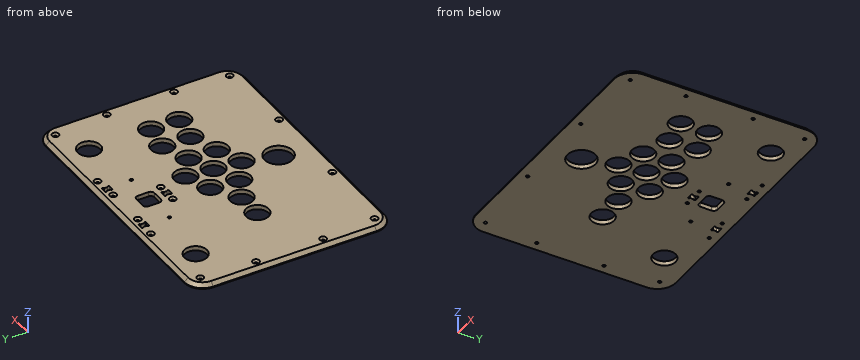
Autodesk Inventor part; units mm, degrees
ref_plane "YZ Plane" through (0, 0, 0) normal (1, 0, 0) x (0, 1, 0)
ref_plane "XZ Plane" through (0, 0, 0) normal (0, 1, 0) x (-1, 0, 0)
ref_plane "XY Plane" through (0, 0, 0) normal (0, 0, 1) x (1, 0, 0)
sketch "Sketch1" plane through (0, 0, 0) normal (0, 0, 1) x (1, 0, 0)
  line L0 (-150, 110) -> (150, 110)
  line L1 (150, 110) -> (150, -110)
  line L2 (150, -110) -> (-150, -110)
  line L3 (-150, -110) -> (-150, 110)
  line L4 (-150, 110) -> (150, -110) construction
  line L5 (150, 110) -> (-150, -110) construction
  point P0 (0, 0)
  dimension "d0" = 300
  dimension "d1" = 220
extrude "Extrusion1" add sketch "Sketch1" along normal blind 5
sketch "Sketch2" plane through (0, 0, 5) normal (0, 0, 1) x (1, 0, 0)
  line L0 (-150, -110) -> (150, -110)
  line L1 (9.7, -35) -> (14.9, 23.8) construction
  line L2 (-12.9, 12.8) -> (37.5, -24) construction
  line L3 (-100, 80) -> (100, 80) construction
  line L4 (150, 110) -> (-150, 110)
  line L5 (-150, 110) -> (-150, -110)
  arc A0 (9.7, -35) -> (-41.8, -4.7) centre (-117.4638, -192.22) ccw
  point P0 (0, 0)
  point P1 (0, -70)
  point P2 (-15.5, -17.6)
  point P3 (-71.3, -4.8)
  point P4 (12.3, -5.6)
  point P5 (39.2, 6.1)
  point P6 (68.8, -13.3)
  point P7 (68.8, 17.7)
  point P8 (98.3, -18.3)
  point P9 (98.3, 12.7)
  point P10 (12.3, -5.6)
  point P11 (0, 80)
  point P12 (-60, 80)
  point P13 (60, 80)
  point P14 (31.5334, -55.5137)
  point P15 (-14.9246, -17.9372)
  dimension "d4" = 40
  dimension "d5" = 15.5
  dimension "d6" = 26.3
  dimension "d7" = 29.5
  dimension "d11" = 52.4
  dimension "d12" = 65.3
  dimension "d13" = 65.2
  dimension "d14" = 9.7
  dimension "d15" = 29.4
  dimension "d16" = 2.6
  dimension "d17" = 26.9
  dimension "d18" = 29.6
  dimension "d19" = 29.5
  dimension "d20" = 1.7
  dimension "d22" = 46
  dimension "d23" = 30.1
  dimension "d24" = 96.7
  dimension "d25" = 91.7
  dimension "d26" = 31
  dimension "d27" = 31
  dimension "d28" = 35
  dimension "d61" = 30
  dimension "d62" = 50
  dimension "d63" = 8.496
  dimension "d64" = 8.496
  dimension "d65" = 40
  dimension "d66" = 40
hole "Hole1" at (0, -70, 5) at (-15.5, -17.6, 5) at (-41.8, -4.7, 5) at (-71.3, -4.8, 5) at (9.7, -35, 5) at (12.3, -5.6, 5) at (37.5, -24, 5) at (39.2, 6.1, 5) at (68.8, -13.3, 5) at (68.8, 17.7, 5) at (98.3, -18.3, 5) at (98.3, 12.7, 5) at (-12.9, 12.8, 5) at (14.9, 23.8, 5) at (-100, 80, 5) at (100, 80, 5) direction (0, 0, -1) diameter 25 end through all
sketch "Sketch5" plane through (0, 0, 5) normal (0, 0, 1) x (1, 0, 0)
  circle A0 centre (0, -70) radius 12.5
  point P0 (0, 0)
hole "Hole2" at (0, -70, 5) direction (0, 0, -1) diameter 31 end through all
sketch "Sketch6" plane through (0, 0, 5) normal (0, 0, 1) x (1, 0, 0)
  line L0 (-35.7, 71.2) -> (35.7, 71.2) construction
  line L1 (150, 110) -> (-150, 110)
  point P0 (0, 0)
  point P1 (0, 71.2)
  dimension "d67" = 71.4
  dimension "d68" = 38.8
hole "Hole3" at (-35.7, 71.2, 5) at (35.7, 71.2, 5) direction (0, 0, -1) diameter 3.4 end through all
fillet "Fillet2" radius 20 4 edges at (-150, 110, 2.5) (-150, -110, 2.5) (150, -110, 2.5) (150, 110, 2.5)
chamfer "Chamfer1" distance 4 angle 45 8 edges at (0, -110, 5) (144.1421, -104.1421, 5) (150, 0, 5) (144.1421, 104.1421, 5) (0, 110, 5) (-144.1421, 104.1421, 5) (-150, 0, 5) (-144.1421, -104.1421, 5)
sketch "Sketch8" plane through (0, 0, 5) normal (0, 0, 1) x (1, 0, 0)
  line L0 (130, 110) -> (-130, 110)
  line L1 (-150, 90) -> (-150, -90)
  line L2 (-130, -110) -> (130, -110)
  line L3 (150, -90) -> (150, 90)
  point P0 (0, 0)
  point P1 (-140, 37)
  point P2 (-50, 100)
  point P3 (-136, 96)
  dimension "d85" = 10
  dimension "d86" = 10
  dimension "d87" = 220
  dimension "d88" = 300
  dimension "d89" = 73
  dimension "d90" = 100
  dimension "d91" = 14
  dimension "d92" = 14
hole "Hole4" at (-140, 37, 5) at (-50, 100, 5) at (-136, 96, 5) direction (0, 0, -1) diameter 3.4 end through all countersink diameter 7.5 countersink angle 90
mirror "Mirror1" about plane through (0, 0, 0) normal (1, 0, 0) of "Hole4"
mirror "Mirror2" about plane through (0, 0, 0) normal (0, 1, 0) of "Hole4", "Mirror1"
sketch "Sketch9" plane through (0, 0, 5) normal (0, 0, 1) x (1, 0, 0)
  line L0 (-6, 83.2) -> (6, 83.2)
  line L1 (10, 79.2) -> (10, 67.2)
  line L2 (6, 63.2) -> (-6, 63.2)
  line L3 (-10, 67.2) -> (-10, 79.2)
  circle A0 centre (-35.7, 71.2) radius 1.7
  circle A1 centre (35.7, 71.2) radius 1.7
  line L4 (-35.7, 71.2) -> (35.7, 71.2) construction
  arc A2 (-6, 83.2) -> (-10, 79.2) centre (-6, 79.2) ccw
  arc A3 (10, 79.2) -> (6, 83.2) centre (6, 79.2) ccw
  arc A4 (-10, 67.2) -> (-6, 63.2) centre (-6, 67.2) ccw
  arc A5 (6, 63.2) -> (10, 67.2) centre (6, 67.2) ccw
  point P0 (0, 0)
  point P1 (-10, 83.2)
  point P2 (10, 63.2)
  point P3 (10, 83.2)
  point P4 (0, 83.2)
  point P5 (0, 71.2)
  point P6 (-10, 73.2)
  dimension "d100" = 20
  dimension "d101" = 20
  dimension "d102" = 2
  dimension "d103" = 4
extrude "Extrusion5" cut sketch "Sketch9" against normal through all contours L0 A3 L1 A5 L2 A4 L3 A2
sketch "Sketch10" plane through (0, 0, 5) normal (0, 0, 1) x (1, 0, 0)
  line L0 (-11.25, 53.2) -> (11.25, 53.2) construction
  circle A0 centre (35.7, 71.2) radius 1.7
  circle A1 centre (-35.7, 71.2) radius 1.7
  circle A2 centre (35.7, 71.2) radius 1.7
  line L1 (-35.7, 71.2) -> (35.7, 71.2) construction
  line L2 (0, 71.2) -> (0, 98.6) construction
  line L3 (-34.4, 98.6) -> (34.4, 98.6) construction
  line L4 (23.15, 98.6) -> (45.65, 98.6) construction
  line L5 (-45.65, 98.6) -> (-23.15, 98.6) construction
  point P0 (0, 0)
  point P1 (0, 53.2)
  dimension "d106" = 22.5
  dimension "d107" = 18
  dimension "d108" = 22.5
  dimension "d109" = 22.5
  dimension "d110" = 27.4
  dimension "d111" = 68.8
hole "Hole5" at (-11.25, 53.2, 5) at (11.25, 53.2, 5) at (23.15, 98.6, 5) at (-23.15, 98.6, 5) direction (0, 0, -1) diameter 3.4 end through all countersink diameter 7.5 countersink angle 90
sketch "Sketch11" plane through (0, 0, 5) normal (0, 0, 1) x (1, 0, 0)
  circle A0 centre (-11.25, 53.2) radius 1.7 construction
  circle A1 centre (11.25, 53.2) radius 1.7 construction
  line L0 (-11.25, 53.2) -> (11.25, 53.2) construction
  circle A2 centre (23.15, 98.6) radius 1.7 construction
  line L1 (23.15, 98.6) -> (45.65, 98.6) construction
  line L2 (-23.15, 98.6) -> (-45.65, 98.6) construction
  line L3 (-2.55, 49.15) -> (2.55, 49.15)
  line L4 (2.55, 49.15) -> (2.55, 57.25)
  line L5 (2.55, 57.25) -> (-2.55, 57.25)
  line L6 (-2.55, 57.25) -> (-2.55, 49.15)
  line L7 (-2.55, 49.15) -> (2.55, 57.25) construction
  line L8 (2.55, 49.15) -> (-2.55, 57.25) construction
  circle A3 centre (-2.55, 50.15) radius 1
  circle A4 centre (2.55, 50.15) radius 1
  circle A5 centre (2.55, 56.25) radius 1
  circle A6 centre (-2.55, 56.25) radius 1
  line L9 (-36.95, 94.55) -> (-31.85, 94.55)
  line L10 (-31.85, 94.55) -> (-31.85, 102.65)
  line L11 (-31.85, 102.65) -> (-36.95, 102.65)
  line L12 (-36.95, 102.65) -> (-36.95, 94.55)
  line L13 (-36.95, 94.55) -> (-31.85, 102.65) construction
  line L14 (-31.85, 94.55) -> (-36.95, 102.65) construction
  circle A7 centre (-36.95, 95.55) radius 1
  circle A8 centre (-31.85, 95.55) radius 1
  circle A9 centre (-31.85, 101.65) radius 1
  circle A10 centre (-36.95, 101.65) radius 1
  line L15 (31.85, 94.55) -> (36.95, 94.55)
  line L16 (36.95, 94.55) -> (36.95, 102.65)
  line L17 (36.95, 102.65) -> (31.85, 102.65)
  line L18 (31.85, 102.65) -> (31.85, 94.55)
  line L19 (31.85, 94.55) -> (36.95, 102.65) construction
  line L20 (36.95, 94.55) -> (31.85, 102.65) construction
  circle A11 centre (31.85, 95.55) radius 1
  circle A12 centre (36.95, 95.55) radius 1
  circle A13 centre (36.95, 101.65) radius 1
  circle A14 centre (31.85, 101.65) radius 1
  circle A15 centre (-23.15, 98.6) radius 1.7
  point P0 (0, 0)
  point P1 (0, 53.2)
  point P2 (-34.4, 98.6)
  point P3 (34.4, 98.6)
  point P4 (31.85, 100.65)
  point P5 (31.85, 96.55)
  point P6 (36.95, 96.55)
  point P7 (36.95, 100.65)
  point P8 (-31.85, 96.55)
  point P9 (-31.85, 100.65)
  point P10 (-36.95, 100.65)
  point P11 (-36.95, 96.55)
  point P12 (-2.55, 55.25)
  point P13 (-2.55, 51.15)
  point P14 (2.55, 51.15)
  point P15 (2.55, 55.25)
  dimension "d121" = 2
  dimension "d124" = 2
  dimension "d127" = 2
  dimension "d119" = 8.1
  dimension "d120" = 5.1
  dimension "d122" = 8.1
  dimension "d123" = 5.1
  dimension "d125" = 8.1
  dimension "d126" = 5.1
  dimension "d130" = 11.25
  dimension "d131" = 11.25
  dimension "d132" = 11.25
extrude "Extrusion6" cut sketch "Sketch11" against normal through all contours A3 L6 A6 L5 A5 L4 A4 L3 | A3 L6 | L6 A3 | A4 L4 | L4 A4 | A6 L6 | L6 A6 | A5 L4 | L4 A5 | A7 L12 A10 L11 A9 L10 A8 L9 | A7 L12 | L12 A7 | A8 L10 | L10 A8 | A10 L12 | L12 A10 | A9 L10 | L10 A9 | A11 L18 A14 L17 A13 L16 A12 L15 | A11 L18 | L18 A11 | A12 L16 | L16 A12 | A14 L18 | L18 A14 | A13 L16 | L16 A13
properties part number "Top Plate Sanwa" material "Polycarbonate, Clear"
Geometry: final body of the model. Coordinates: model frame, mm. Give positions to 0.01 mm unless a question says otherwise; leave off trailing zeros. Loops run counter-clockwise (first coordinate to the right, second up) from the corner with the lowest first, then second, coordinate; pieces in that order, holes last. Notation, with made-up numbers: (32, -38.75) -> (62, -38.75) arc R22 ccw to (62, -20.75) -> close; hole circle Ø3 at (-6.75, 9.5). An arc over 180 degrees is marked (long way). Use one line per item in the form item = value.
Item 1: Pin query (flat end, axial travel): P1, Ø1.5, axis at y = -47, z = 3, coming from the -X side; P2, Ø3, axis at x = -50, y = -100, coming from the +Z side; P3, Ø1.5, axis at x = 28, z = 2, coming from the +Y side; P4, Ø1.5, axis at x = -17.5, z = 4, coming from the +Y side. Return the tip coordinate at first contact, or that it passes through.
A:
P1 = -148.75
P2 = through
P3 = 109.75
P4 = 107.75
Item 2: Section query B-B on x = 92.5. Output: boundary loops of the cut face in (y, z).
A:
outline = (-110, 0) -> (-29.37, 0) -> (-29.37, 5) -> (-106, 5) -> (-110, 1) -> close; (-7.23, 0) -> (1.63, 0) -> (1.63, 5) -> (-7.23, 5) -> close; (23.77, 0) -> (70, 0) -> (70, 5) -> (23.77, 5) -> close; (90, 0) -> (110, 0) -> (110, 1) -> (106, 5) -> (90, 5) -> close
Item 3: Section query A-A on x = -41.8. Output: boundary loops of the cut face in (y, z), and give its area (3 significant figures).
A:
outline = (-110, 0) -> (-17.2, 0) -> (-17.2, 5) -> (-106, 5) -> (-110, 1) -> close; (7.8, 0) -> (110, 0) -> (110, 1) -> (106, 5) -> (7.8, 5) -> close
area = 959 mm^2
Item 4: Line query: probe 1 along X at (y, z) = (-38, 2.4); probe 2 along Y at (x, z) = (60.5, 4.7); probe 3 along Y at (x, z) = (60, 2.8). Output: solid intervals per line, ascending.
A:
probe_1 = -148.6 to -141.37, -138.63 to -2.43, 21.83 to 138.63, 141.37 to 148.6
probe_2 = -106.3 to -22.65, -3.95 to 8.35, 27.05 to 106.3
probe_3 = -108.2 to -22.18, -4.42 to 8.82, 26.58 to 108.2
